Could you check a few things on this model? Use its own coordinates, in mm. Face numbers are marked on the shaded views. A direction names the side the tool comes from. Give positions to 0.01 mm unless a question says otherwise; leave off trailing zeros. Write each loop counter-clockwise with the first axis right and the second up, starting at its lowest first coordinate (ties: lowest second). Pieces come first, ordered by that corner, then holes. Notation, with made-up numbers: (22, 86.25) - (72, 86.25) arc R38 cw to (72, 125.25) - close; hole circle Ø10 at (63.5, -5.75). An arc over 180 degrees is marked (long way). Write item = value, one per line.
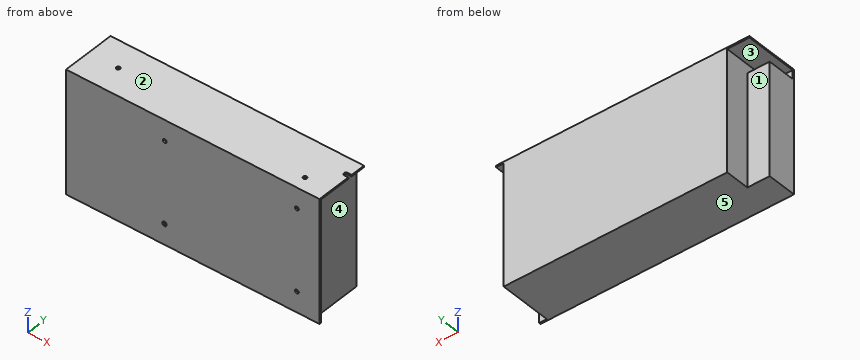
from build123d import *

# Parameters (mm, degrees)
SZKIC1_W                    = 200
SZKIC1_H                    = 97
DODANIE_WYCI_GNI_CIE1_DEPTH = 1.25
SZKIC2_W                    = 200
SZKIC2_H                    = 1.25
DODANIE_WYCI_GNI_CIE2_DEPTH = 42.6
SZKIC4_R                    = 1.5
SZKIC4_R_2                  = 1.746235722
WYTNIJ_WYCI_GNI_CIE1_DEPTH  = 1.25
SZKIC5_W                    = 182.404557989
SZKIC5_H                    = 95.75
DODANIE_WYCI_GNI_CIE3_DEPTH = 41.35
SZKIC6_W                    = 17.595442011
SZKIC6_H                    = 88.898428246
DODANIE_WYCI_GNI_CIE4_DEPTH = 22
SZKIC3_R                    = 1.5
WYTNIJ_WYCI_GNI_CIE2_DEPTH  = 1.25
SZKIC7_W                    = 95.75
SZKIC7_H                    = 41.35
WYTNIJ_WYCI_GNI_CIE3_DEPTH  = 6


with BuildPart() as part:
    # Szkic1 → Dodanie-wyciągnięcie1 (new body)
    with BuildSketch(Plane(origin=(0, 0, 0), x_dir=(1, 0, 0), z_dir=(0, 1, 0))):
        with Locations((39.453125, 6.3828125)):
            Rectangle(SZKIC1_W, SZKIC1_H)
    extrude(amount=DODANIE_WYCI_GNI_CIE1_DEPTH)

    # Szkic2 → Dodanie-wyciągnięcie2 (add)
    with BuildSketch(Plane.XZ):
        with Locations((39.453125, 41.4921875)):
            Rectangle(SZKIC2_W, SZKIC2_H)
    extrude(amount=-DODANIE_WYCI_GNI_CIE2_DEPTH)

    # Szkic4 → Wytnij-wyciągnięcie1 (cut)
    with BuildSketch(Plane.XZ):
        with Locations(Location((121.653125, -38.6328125, 0), (0, 0, 270))):
            Circle(SZKIC4_R)
        with Locations(Location((121.653125, 25.8671875, 0), (0, 0, 270))):
            Circle(SZKIC4_R)
        with Locations(Location((17.106889278, -38.6328125, 0), (0, 0, 270))):
            Circle(SZKIC4_R_2)
        with Locations(Location((17.353125, 25.8671875, 0), (0, 0, 270))):
            Circle(SZKIC4_R)
    extrude(amount=-WYTNIJ_WYCI_GNI_CIE1_DEPTH, mode=Mode.SUBTRACT)

    # Szkic5 → Dodanie-wyciągnięcie3 (add)
    with BuildSketch(Plane(origin=(0, 1.25, 0), x_dir=(1, 0, 0), z_dir=(0, 1, 0))):
        with Locations((48.250846005, 7.0078125)):
            Rectangle(SZKIC5_W, SZKIC5_H)
    extrude(amount=DODANIE_WYCI_GNI_CIE3_DEPTH)

    # Szkic6 → Dodanie-wyciągnięcie4 (add)
    with BuildSketch(Plane(origin=(0, 1.25, 0), x_dir=(1, 0, 0), z_dir=(0, 1, 0))):
        with Locations((-51.749153995, 10.433598377)):
            Rectangle(SZKIC6_W, SZKIC6_H)
    extrude(amount=DODANIE_WYCI_GNI_CIE4_DEPTH)

    # Szkic3 → Wytnij-wyciągnięcie2 (cut)
    with BuildSketch(Plane.XY.offset(42.1171875)):
        with Locations((119.153125, 10.8)):
            Circle(SZKIC3_R)
        with Locations((-36.946875, 21.3)):
            Circle(SZKIC3_R)
        with BuildLine():
            Line((136.353125, 30.8), (139.453125, 30.8))
            Line((139.453125, 30.8), (139.453125, 27.6))
            Line((139.453125, 27.6), (136.353125, 27.6))
            ThreePointArc((136.353125, 27.6), (134.753125, 29.2), (136.353125, 30.8))
        make_face()
    extrude(amount=-WYTNIJ_WYCI_GNI_CIE2_DEPTH, mode=Mode.SUBTRACT)

    # Szkic7 → Wytnij-wyciągnięcie3 (cut)
    with BuildSketch(Plane(origin=(139.453125, 0, 0), x_dir=(0, 0, -1), z_dir=(1, 0, 0))):
        with Locations((7.0078125, 21.925)):
            Rectangle(SZKIC7_W, SZKIC7_H)
    extrude(amount=-WYTNIJ_WYCI_GNI_CIE3_DEPTH, mode=Mode.SUBTRACT)


solid = part.part
1. If we section it at B-B, the plane z = -19.5: Please give me the cut outline in (x, y).
Filled sheet:
outline = (-60.55, 0) - (139.45, 0) - (139.45, 1.25) - (133.45, 1.25) - (133.45, 42.6) - (-42.95, 42.6) - (-42.95, 23.25) - (-60.55, 23.25) - close
2. If we section it at A-A, the plane y = 39: Please give me the cut outline in (x, z), and give its area (3 significant figures).
Filled sheet:
outline = (-60.55, 40.87) - (-42.95, 40.87) - (-42.95, -54.88) - (133.45, -54.88) - (133.45, 40.87) - (139.45, 40.87) - (139.45, 42.12) - (-60.55, 42.12) - close
area = 17,100 mm2
3. Which directions (+Z, -Z, +X, -X, +Y, -Y) give clear straight access to the entire face, cutting with the end or side of a thin tool? Please do the marked faces 1, 2, 3, 4 and 5.
Filled sheet:
face_1 = -Z, -X, +Y
face_2 = +Z, +X, -X, +Y, -Y
face_3 = -X, +Y
face_4 = -Z, +X, +Y
face_5 = -Z, +X, -X, +Y, -Y
4. For pin 1 (0.9 mm diameter, centred on x = -37.5, y = 22, fed in from +Z); pin 2 (1.8 mm diameter, centred on x = 135.5, y = 32, fed in from -Z); pin 3 (4 mm diameter, centred on x = 17.35, z = 25.87, fed in from -Y); pin 4 (1.5 mm diameter, centred on y = 17.5, z = -26.5, fed in from +X), each with a flat end and sliding along its axis, tell me the tip position at first contact or that it passes through.
Filled sheet:
pin_1 = 40.87
pin_2 = 40.87
pin_3 = 0
pin_4 = 133.45
5. I need wall thicknesses on line 1 (Z direction, x = -45, y = 15); line 2 (X direction, y = 26.5, z = 10); line 3 (X direction, y = 9.5, z = -13.5). Which ranges of each line are inside material? Lowest first, please.
Filled sheet:
line_1 = -54.88 to 34.02, 40.87 to 42.12
line_2 = -42.95 to 133.45
line_3 = -60.55 to 133.45
